The drawing under review shows one solid part. Ordinate dimensions are in mm from its lowest x, y, z. Round coordinates to 2 decimals unless told otherwise and drop trailing zeros. Write each loop counter-clockwise with the first axis right and the second up, starting at its lowest first coordinate (ties: lowest second). Pieces come first, ordered by that corner, then holes. Notation, with made-up numbers: (-34, 70) -> (-25, 70) arc R20 cw to (-25, 79) -> close; hole circle Ø6 at (-14, 61). An arc over 180 degrees is marked (long way). Answer in a Markdown table with one row per item. Add a question column.
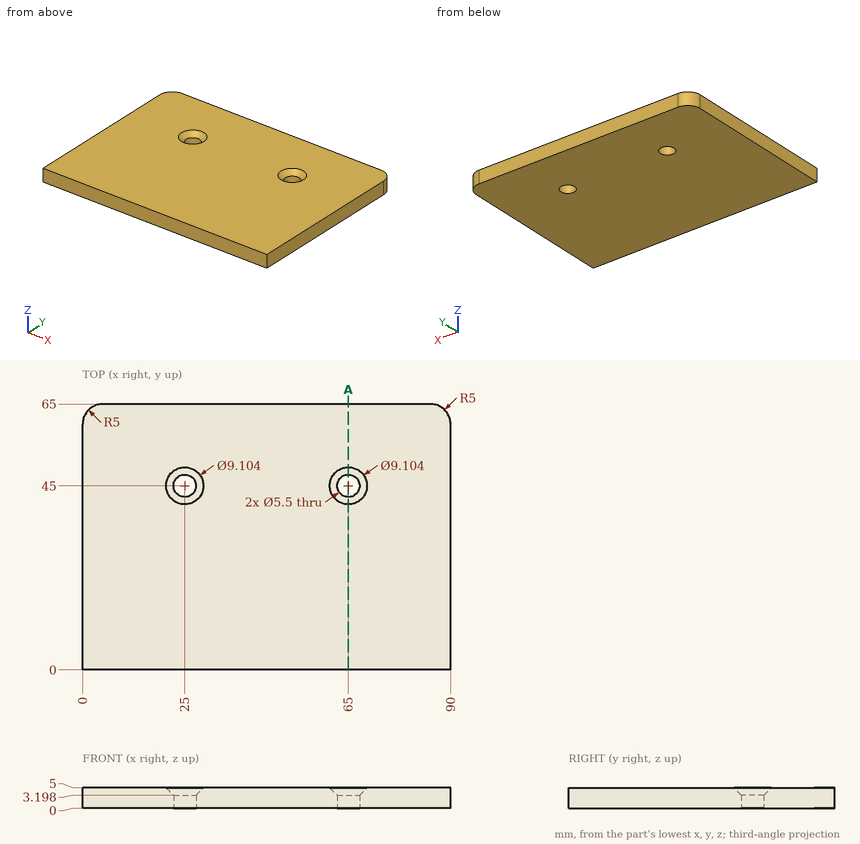
1. For L1, parallel to Y at x = 65, z = 1.2; L2, parallel to X at y = 60.5, z = 2.55 (1 decimal); L3, parallel to Z at x = 64, y = 48.5, list the stretches that pass through material, from the lowest coordinate up.
2. Insertion check: pin 1 Ø4.5 at (x, y) = (65, 45) entering from +Z; pin 2 Ø6.5 at (x, y) = (25, 45) entering from +Z. Each pin has a flat end and moves straight along its axis. Give the tip position at first contact, or say it passes through.
3. Add section A-A on x = 65. Write out the cut boundary in (y, z).
Filled in:
| question | item | result |
|---|---|---|
| 1 | L1 | 0 to 42.25, 47.75 to 65 |
| 1 | L2 | 0 to 90 |
| 1 | L3 | 0 to 4.09 |
| 2 | pin 1 | through |
| 2 | pin 2 | z = 3.7 |
| 3 | outline | (0, 0) -> (42.25, 0) -> (42.25, 3.2) -> (40.45, 5) -> (0, 5) -> close; (47.75, 0) -> (65, 0) -> (65, 5) -> (49.55, 5) -> (47.75, 3.2) -> close |
